The listing builds one solid part. Answer for the finished solid, in the listing's coordinates (mm). Face numbers are marked on the shaded views. A direction names the side the tool comes from. Round coordinates to 2 decimals unless told otherwise and drop trailing zeros. Loops run counter-clockwise (first coordinate to the right, second up) from the corner with the lowest first, then second, coordinate; pieces in that order, holes last. Notation, with made-up numbers: (89.25, 74) -> (120.25, 74) arc R12 ccw to (120.25, 86) -> close; hole circle Ø8 at (-25.5, 69.25). An arc over 180 degrees is marked (long way). One line per question, with ' | ' between items.
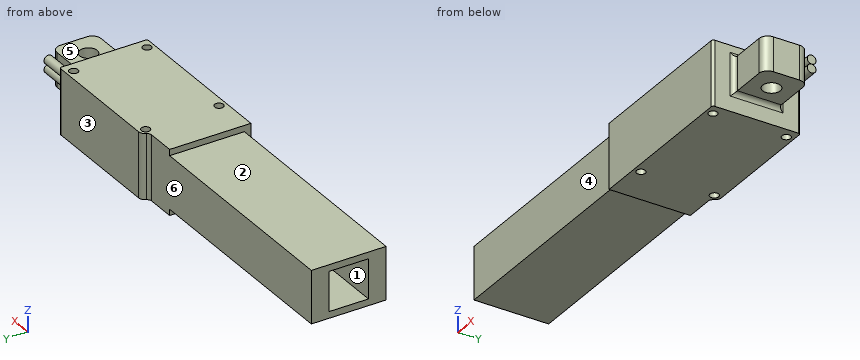
from build123d import *

# Parameters (mm, degrees)
BOSS_EXTRU_1_DEPTH      = 14.8
BOSS_EXTRU_2_START      = -2.6000000000000005
ESQUISSE2_R             = 2.000000000000003
BOSS_EXTRU_2_DEPTH      = 7.8
BOSS_EXTRU_3_START      = -1.4
BOSS_EXTRU_3_DEPTH      = 12
ENL_V_MAT_EXTRU_1_DEPTH = 50
CONG_1_R                = 1
CONG_2_R                = 1
ESQUISSE10_R            = 1.0000000000000018
ENL_V_MAT_EXTRU_2_DEPTH = 73.14603246194486
CONG_3_R                = 0.5
ESQUISSE11_R            = 1.0000000000000013
ESQUISSE11_R_2          = 0.9999999999999998
BOSS_EXTRU_5_DEPTH      = 8


with BuildPart() as part:
    # Esquisse1 → Boss.-Extru.1 (new body)
    with BuildSketch(Plane.XY):
        Polygon((-18.700000000000003, 10), (18.699999999999996, 10), (18.699999999999996, -10), (-18.7, -10), align=None)
    extrude(amount=BOSS_EXTRU_1_DEPTH)

    # Esquisse2 → Boss.-Extru.2 (add)
    with BuildSketch(Plane.XY.offset(14.8).offset(BOSS_EXTRU_2_START)):
        with BuildLine():
            Line((29.5, -3.0000000000000004), (29.5, 3.0000000000000004))
            ThreePointArc((29.5, 3.0000000000000004), (28.914213562373092, 4.414213562373096), (27.499999999999996, 4.999999999999998))
            Line((27.499999999999996, 5), (19.699999999999996, 5))
            ThreePointArc((19.699999999999996, 5.000000000000001), (18.99289321881345, 5.292893218813453), (18.699999999999996, 6))
            Line((18.699999999999996, 6), (18.699999999999996, 5))
            Line((18.699999999999996, 5.000000000000001), (18.699999999999996, -4.999999999999999))
            Line((18.699999999999996, -5), (18.699999999999996, -6))
            ThreePointArc((18.699999999999996, -6), (18.99289321881345, -5.292893218813453), (19.699999999999996, -5.000000000000001))
            Line((19.699999999999996, -5), (27.499999999999996, -5))
            ThreePointArc((27.499999999999996, -4.999999999999999), (28.914213562373096, -4.414213562373097), (29.5, -3.0000000000000004))
        make_face()
        with Locations((24.099999999999998, 0)):
            Circle(ESQUISSE2_R, mode=Mode.SUBTRACT)
    extrude(amount=-BOSS_EXTRU_2_DEPTH)

    # Esquisse4 → Boss.-Extru.3 (add)
    with BuildSketch(Plane.XY.offset(14.8).offset(BOSS_EXTRU_3_START)):
        Polygon((-69.9, 8.499999999999998), (-18.700000000000003, 8.499999999999998), (-18.700000000000003, -8.5), (-69.9, -8.499999999999998), align=None)
    extrude(amount=-BOSS_EXTRU_3_DEPTH)

    # Esquisse7 → Enlèv. mat.-Extru.1 (cut)
    with BuildSketch(Plane.ZY.offset(69.9)):
        Polygon((2.9000000000000026, 4.5), (11.9, 4.5), (11.900000000000004, -4.5), (2.9000000000000044, -4.5), align=None)
    extrude(amount=-ENL_V_MAT_EXTRU_1_DEPTH, mode=Mode.SUBTRACT)

    # Congé1
    cong_1_edges = [part.edges().sort_by_distance(p)[0] for p in [
        (18.699999999999996, 0, 4.4),
    ]]
    fillet(cong_1_edges, radius=CONG_1_R)

    # Congé2
    cong_2_edges = [part.edges().sort_by_distance(p)[0] for p in [
        (18.699999999999996, 0, 12.2),
    ]]
    fillet(cong_2_edges, radius=CONG_2_R)

    # Esquisse10 → Enlèv. mat.-Extru.2 (cut, through all)
    with BuildSketch(Plane.XY.offset(14.8)):
        with Locations((16.2, 8.35)):
            Circle(ESQUISSE10_R)
        with Locations((-9.800000000000002, 8.349999999999994)):
            Circle(ESQUISSE10_R)
        with Locations(Location((-9.80000000000001, -8.349999999999994, 0), (0, 0, 180))):
            Circle(ESQUISSE10_R)
        with Locations(Location((16.19999999999997, -8.35, 0), (0, 0, 180))):
            Circle(ESQUISSE10_R)
        with BuildLine():
            Line((-18.700000000000003, 8.499999999999998), (-12.187467277262673, 8.499999999999998))
            ThreePointArc((-12.187467277262673, 8.499999999999998), (-11.655472100663742, 8.653252616138984), (-11.286536229239028, 9.066037735849054))
            ThreePointArc((-11.286536229239028, 9.066037735849054), (-10.677792041388242, 9.747133183370671), (-9.800000000000002, 10))
            Line((-9.800000000000002, 10), (-18.700000000000003, 10))
            Line((-18.700000000000003, 10), (-18.700000000000003, 8.499999999999998))
        make_face()
    extrude(amount=-ENL_V_MAT_EXTRU_2_DEPTH, mode=Mode.SUBTRACT)

    # Congé3
    cong_3_edges = [part.edges().sort_by_distance(p)[0] for p in [
        (18.699999999999996, -10, 7.4),
        (18.699999999999996, 10, 7.4),
    ]]
    fillet(cong_3_edges, radius=CONG_3_R)

    # Esquisse11 → Boss.-Extru.5 (add)
    with BuildSketch(Plane(origin=(18.699999999999996, 0, 0), x_dir=(0, 0, -1), z_dir=(1, 0, 0))):
        with Locations(Location((-11.821599718382592, 7.5, 0), (0, 0, 180))):
            Circle(ESQUISSE11_R)
        with Locations(Location((-9.811599718382592, 7.5, 0), (0, 0, 180))):
            Circle(ESQUISSE11_R_2)
    extrude(amount=BOSS_EXTRU_5_DEPTH)


solid = part.part
Q1. A cutting plane is placed at C-C on z = 6. Give the vertices of the cut face in (x, y).
Numbers:
outline: (-69.9, -8.5) -> (-18.7, -8.5) -> (-18.7, -10) -> (18.2, -10) arc R0.5 ccw to (18.7, -9.5) -> (18.7, -6) arc R1 cw to (19.7, -5) -> (27.5, -5) arc R2 ccw to (29.5, -3) -> (29.5, 3) arc R2 ccw to (27.5, 5) -> (19.7, 5) arc R1 cw to (18.7, 6) -> (18.7, 9.5) arc R0.5 ccw to (18.2, 10) -> (-9.8, 10) arc R1.65 ccw to (-11.29, 9.07) arc R1 cw to (-12.19, 8.5) -> (-69.9, 8.5) -> (-69.9, 4.5) -> (-19.9, 4.5) -> (-19.9, -4.5) -> (-69.9, -4.5) -> close; hole circle Ø2 at (-9.8, -8.35); hole circle Ø2 at (-9.8, 8.35); hole circle Ø2 at (16.2, -8.35); hole circle Ø2 at (16.2, 8.35); hole circle Ø4 at (24.1, 0)
Q2. A cutting plane is placed at A-A on x = 16.2. Give the vertices of the cut face in (y, z), plus the area to 3 significant figures.
Numbers:
outline: (-10, 0) -> (-9.35, 0) -> (-9.35, 14.8) -> (-10, 14.8) -> close; (-7.35, 0) -> (7.35, 0) -> (7.35, 14.8) -> (-7.35, 14.8) -> close; (9.35, 0) -> (10, 0) -> (10, 14.8) -> (9.35, 14.8) -> close | area: 237 mm^2
Q3. Find the intervals of material crossed by line 1 (Y direction, x = 16.2, z = 4.5); line 2 (Z direction, x = -42.5, y = -3.25); line 3 (Y direction, x = -57, z = 7.25), in increasing order. Write a range as from..to.
Numbers:
line 1: -10..-9.35, -7.35..7.35, 9.35..10 | line 2: 1.4..2.9, 11.9..13.4 | line 3: -8.5..-4.5, 4.5..8.5
Q4. For a pull along Z with two mould halves and no side action, classify the marked faces 1, 2 and 3 as pulls with the +Z half, pulls with the -Z half, needs draft (parallel to the pull), parting line crosses it, or undercut.
Numbers:
face 1: undercut | face 2: pulls with the +Z half | face 3: needs draft
Q5. Given pin 1 Ø6 at (x, z) = (23.5, 9.5) entering from -Y; pin 2 Ø7 at (x, z) = (-41, 8.5) entering from -Y; pin 3 Ø0.6 at (y, z) = (7.5, 11.5) entering from +X, each flat-ended and moving along its own axis, determine where each tip first touches the part or whether it passes through.
Numbers:
pin 1: y = -5 | pin 2: y = -8.5 | pin 3: x = 26.7
Q6. A cutting plane is placed at B-B on y = 0. Give the vertices of the cut face in (x, z).
Numbers:
outline: (-69.9, 1.4) -> (-18.7, 1.4) -> (-18.7, 0) -> (18.7, 0) -> (18.7, 3.4) arc R1 cw to (19.7, 4.4) -> (22.1, 4.4) -> (22.1, 12.2) -> (19.7, 12.2) arc R1 cw to (18.7, 13.2) -> (18.7, 14.8) -> (-18.7, 14.8) -> (-18.7, 13.4) -> (-69.9, 13.4) -> (-69.9, 11.9) -> (-19.9, 11.9) -> (-19.9, 2.9) -> (-69.9, 2.9) -> close; (26.1, 4.4) -> (29.5, 4.4) -> (29.5, 12.2) -> (26.1, 12.2) -> close
Q7. A cutting plane is placed at D-D on x = -45. Give the vertices of the cut face in (y, z), plus the area to 3 significant figures.
Numbers:
outline: (-8.5, 1.4) -> (8.5, 1.4) -> (8.5, 13.4) -> (-8.5, 13.4) -> close; hole (-4.5, 2.9) -> (4.5, 2.9) -> (4.5, 11.9) -> (-4.5, 11.9) -> close | area: 123 mm^2
Q8. For the marked faces 4, 5 and 6, determine the directions among +Z, -Z, +X, -X, +Y, -Y from which every point of the face is accessible in a straight line to the end or side of a thin tool.
Numbers:
face 4: +Z, -Z, -X, -Y | face 5: +Z, +X, -Y | face 6: +Z, -Z, -X, +Y
